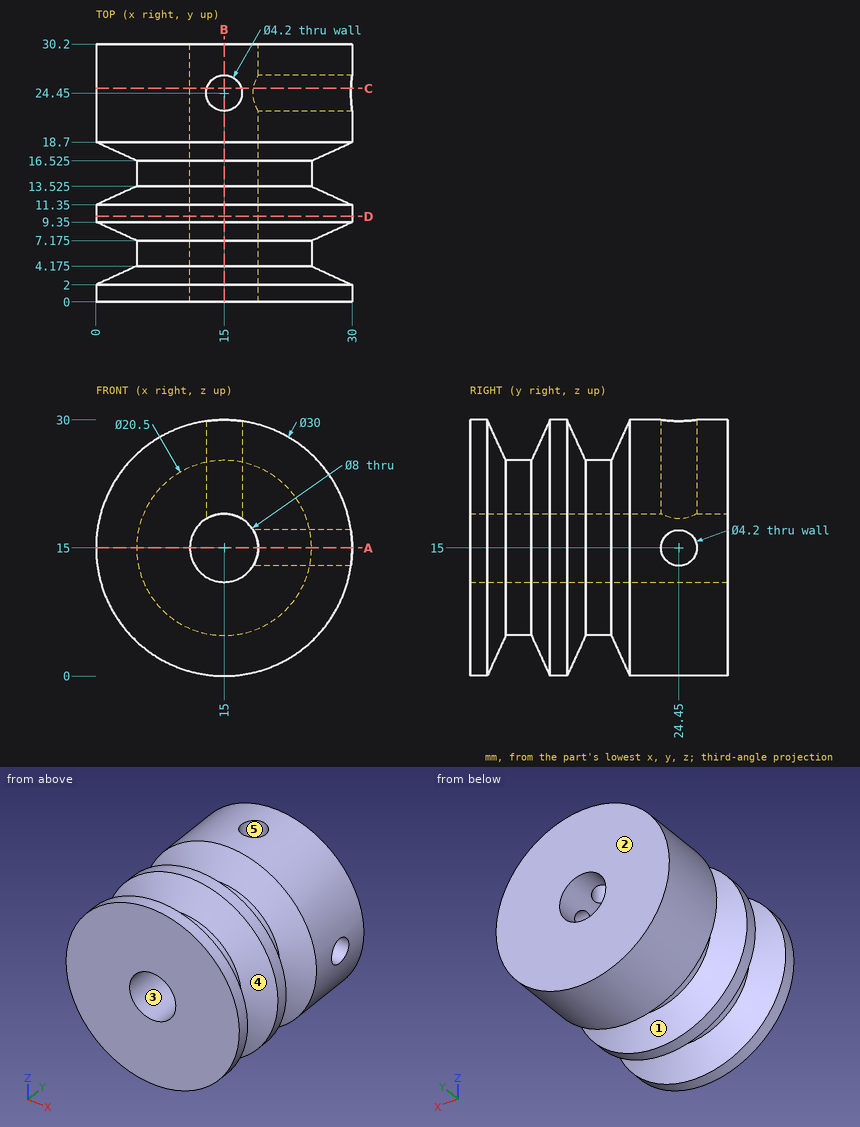
Geometry check sheet. Reference: drawing and pictorial views, mm from the part's lowest x, y, z. A direction names the side the tool comes from. Give positions to 0.01 mm unless a question says otherwise; leave off trailing zeros. Loops run counter-clockwise (first coordinate to the right, second up) from the corner with the lowest first, then second, coordinate; pieces in that order, holes last. Notation, with made-up numbers: (-38.75, 63.25) - (-21.75, 63.25) arc R16 cw to (-21.75, 85.25) - close; hole circle Ø6 at (60.5, 38). An arc over 180 degrees is marked (long way). One line per question, with ' | ' between items. Start each with the question number.
1. Cross-section at B-B, the plane x = 15. Enter the section's corners in (y, z) (3 decimals), plus the area to 3 significant figures.
2. Draft check along Z on the marked faces 3, 4 and 5. Enter one of: released by +Z, released by -Z, zero draft, split by the parting line, or undercut.
3. Material ranges on line 1 along Y through (x, z) = (23, 15); line 2 along Y through (x, z) = (25.5, 6); line 3 along Y through (x, z) = (28, 22), recorded low to high. Write a range as [from, to].
4. Set-up check for the marked faces 1 and 2: record each of +Z, -Z, +X, -X, +Y, -Y from which the full face is reachable in a straight line by a thin tool's end or side.
5. Gauge pin test, flat ends, axial feed: pin 1 Ø9 at (x, z) = (15, 15) entering from +Y; pin 2 Ø1 at (y, z) = (10, 17) entering from -X; pin 3 Ø1 at (x, y) = (16, 17) entering from -Z; pin 4 Ø8 at (x, y) = (4.5, 6.5) entering from +Z. Record the tip position at first contact, or that the pin passes through.
6. Cross-section at A-A, the plane z = 15. Enter the section's corners in (x, y) (3 decimals).
7. Cross-section at D-D, the plane y = 10. Enter the section's corners in (x, z), plus the area to 3 significant figures.
8. Cross-section at C-C, the plane y = 25. Enter the section's corners in (x, z).
Check result:
1) outline: (0, 0) - (2, 0) - (4.175, 4.75) - (7.175, 4.75) - (9.35, 0) - (11.35, 0) - (13.525, 4.75) - (16.525, 4.75) - (18.7, 0) - (30.2, 0) - (30.2, 11) - (0, 11) - close; (0, 19) - (22.35, 19) - (22.35, 30) - (18.7, 30) - (16.525, 25.25) - (13.525, 25.25) - (11.35, 30) - (9.35, 30) - (7.175, 25.25) - (4.175, 25.25) - (2, 30) - (0, 30) - close; (26.55, 19) - (30.2, 19) - (30.2, 30) - (26.55, 30) - close | area: 520 mm2
2) face 3: undercut | face 4: split by the parting line | face 5: zero draft
3) line 1: y = [0, 22.35], [26.55, 30.2] | line 2: y = [0, 2.54], [8.81, 11.89], [18.16, 30.2] | line 3: y = [0, 2.11], [9.24, 11.46], [18.59, 30.2]
4) face 1: none | face 2: +Z, -Z, +X, -X, +Y
5) pin 1: stops at y = 30.2 | pin 2: stops at x = 0.08 | pin 3: stops at z = 2.66 | pin 4: stops at z = 27.88
6) outline: (0, 0) - (11, 0) - (11, 30.2) - (0, 30.2) - (0, 18.7) - (4.75, 16.525) - (4.75, 13.525) - (0, 11.35) - (0, 9.35) - (4.75, 7.175) - (4.75, 4.175) - (0, 2) - close; (19, 0) - (30, 0) - (30, 2) - (25.25, 4.175) - (25.25, 7.175) - (30, 9.35) - (30, 11.35) - (25.25, 13.525) - (25.25, 16.525) - (30, 18.7) - (30, 22.35) - (19, 22.35) - close; (19, 26.55) - (30, 26.55) - (30, 30.2) - (19, 30.2) - close
7) outline: circle Ø30 at (15, 15); hole circle Ø8 at (15, 15) | area: 657 mm2
8) outline: (12.97, 18.45) - (12.97, 29.86) arc R15 ccw (long way) to (29.86, 12.97) - (18.45, 12.97) arc R4 cw (long way) to start; (17.03, 18.45) arc R4 cw to (18.45, 17.03) - (29.86, 17.03) arc R15 ccw to (17.03, 29.86) - close
